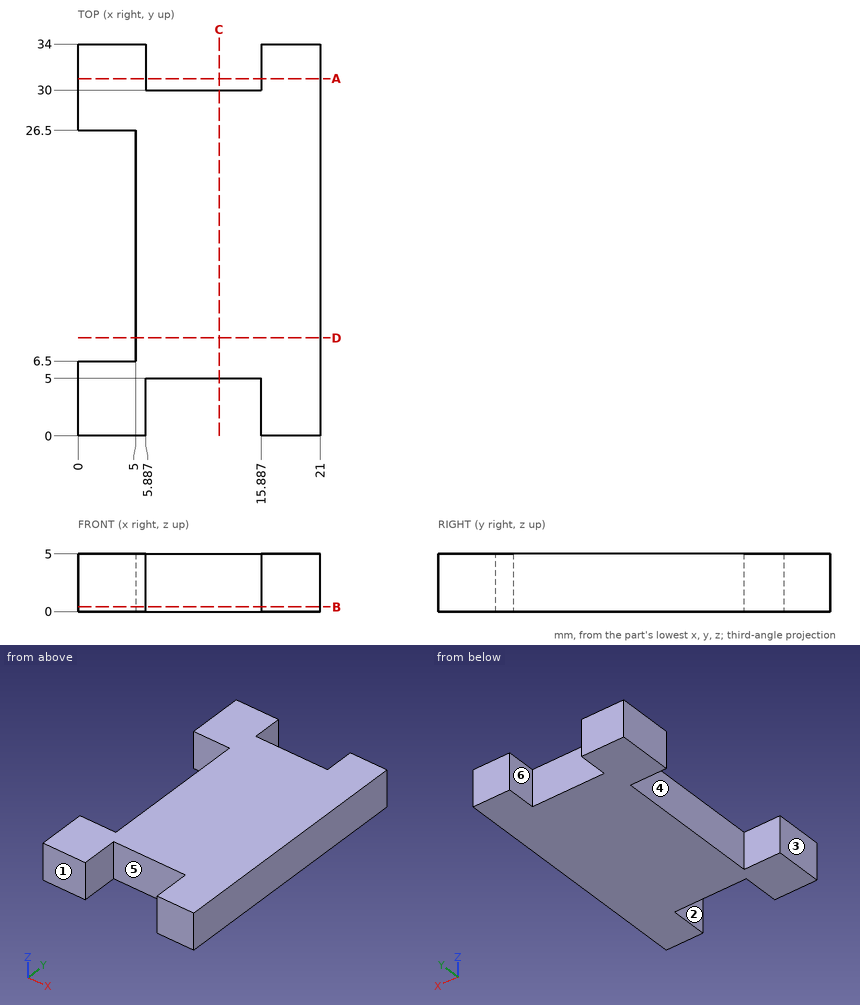
Source: three-view drawing plus pictorial views. Frame: mm from the lowest corner of the part. A direction names the side the tool comes from. Give positions to 0.01 mm unless a question says otherwise; leave off trailing zeros. Order: outer loops, then holes, each group sorted by start corner. A loop starts at its lowest first (then second) coordinate and runs counter-clockwise, first axis right, second up. Notation, with made-up numbers: M -15.75,68.25 L 42.25,68.25 A27 ccw 42.25,97.25 Z; hole C 22.25,42.25 d9. An arc over 180 degrees is marked long. Return JSON: item names as keys, results as strings.
Item 1: Cut plane A-A (y = 31). Return loops of the section in (x, z), then the cut area to 3 significant figures.
Solutions:
{"outline": "M 0,0 L 5.89,0 L 5.89,5 L 0,5 Z; M 15.89,0 L 21,0 L 21,5 L 15.89,5 Z", "area": "55.0 mm^2"}
Item 2: First-contact query: P1, Ø3, axis at y = 31.5, z = 2, coming from the -X side; P2, Ø1, axis at x = 6.5, z = 2, coming from the -Y side; P3, Ø2.5, axis at y = 17.5, z = 2, coming from the -X side. Flat tips, straight axial feed; report the tip coordinate or a pass-through.
Solutions:
{"P1": "x = 0", "P2": "y = 5", "P3": "x = 5"}
Item 3: Cut plane D-D (y = 8.5). Return loops of the section in (x, z), then the cut area to 3 significant figures.
Solutions:
{"outline": "M 5,0 L 21,0 L 21,5 L 5,5 Z", "area": "80.0 mm^2"}
Item 4: Ray query, probe 1 along X at (y, z) = (2, 1.55); probe 2 along Y at (x, z) = (4.25, 1.75); probe 3 along X at (y, z) = (16.5, 3.8). Return the intervals inside material, ascending.
Solutions:
{"probe 1": "0 to 5.89, 15.89 to 21", "probe 2": "0 to 6.5, 26.5 to 34", "probe 3": "5 to 21"}
Item 5: Cut plane C-C (x = 12.25). Return loops of the section in (y, z).
Solutions:
{"outline": "M 5,0 L 30,0 L 30,5 L 5,5 Z"}
Item 6: Cut plane B-B (z = 0.4). Return loops of the section in (x, y), then the cut area to 3 significant figures.
Solutions:
{"outline": "M 0,0 L 5.89,0 L 5.89,5 L 15.89,5 L 15.89,0 L 21,0 L 21,34 L 15.89,34 L 15.89,30 L 5.89,30 L 5.89,34 L 0,34 L 0,26.5 L 5,26.5 L 5,6.5 L 0,6.5 Z", "area": "524 mm^2"}
Item 7: Access query for the marked faces 4, 5 and 6. Directions: +Z, -Z, +X, -X, +Y, -Y. A direction counts if a zero-diameter tool reaches every point of the face in a straight line with its end or side. Return the directions, or none.
Solutions:
{"face 4": "+Z, -Z, -X", "face 5": "+Z, -Z, -Y", "face 6": "+Z, -Z, +Y"}
Item 8: Pull-direction query (X, two-part tool) for the marked faces 1, 2 and 3; classes: +X half, -X half, draft (parallel to the pull), parting line (faces both ways), or undercut.
Solutions:
{"face 1": "draft", "face 2": "undercut", "face 3": "-X half"}
